Answer from the drawing. Dimensions are ordinates in mm from the lowest x, y and z of the part. A direction names the side the tool comes from. Round coordinates to 2 decimals unless told otherwise and drop trailing zeros. Order: outer loops, then holes, each group sorted by start corner. A loop starts at its lowest first (then second) coordinate and runs counter-clockwise, first axis right, second up. Notation, with made-up numbers: (88.25, 69) - (140.25, 69) arc R22 ccw to (140.25, 83) - close; hole circle Ø3 at (13, 16.25). An arc over 180 degrees is marked (long way). One line per question, with ' | ' between items. Start each with the question number.
1) Flat-ended cylindrical pins translate along their axes: pin 1 (13.5 mm diameter, centred on x = 349, z = 53.5, fed in from -Y); pin 2 (1.5 mm diameter, centred on x = 227, y = 19.5, fed in from -Z); pin 3 (2 mm diameter, centred on x = 191.5, z = 192.5, fed in from +Y). Find the tip coordinate at first contact, or state that the pin passes through.
2) The part is cut by section D-D, the plane x = 162. Give the vertices of the cut face in (y, z), plus the area to 3 significant figures.
3) The mould has two halves that part along Z. Classify the marked faces 3, 4 and 5: pulls with the +Z half, pulls with the -Z half, needs draft (parallel to the pull), parting line crosses it, or undercut.
4) The part is cut by section C-C, the plane z = 170.5. Give the vertices of the cut face in (x, y), plus the area to 3 significant figures.
5) For the marked faces 1 and 2, determine the directions among +Z, -Z, +X, -X, +Y, -Y from which every point of the face is accessible in a straight line to the end or side of a thin tool.
6) Straight lines are drawn through the part: line 1 (Z direction, x = 50, y = 14.5); line 2 (Z direction, x = 200, y = 20); line 3 (X direction, y = 15, z = 369). For each, find the intervals that lie inside material, in ascending order. Write a range as from..to.
7) The part is cut by section A-A, the plane y = 8.5. Give the vertices of the cut face in (x, z), plus the area to 3 significant figures.
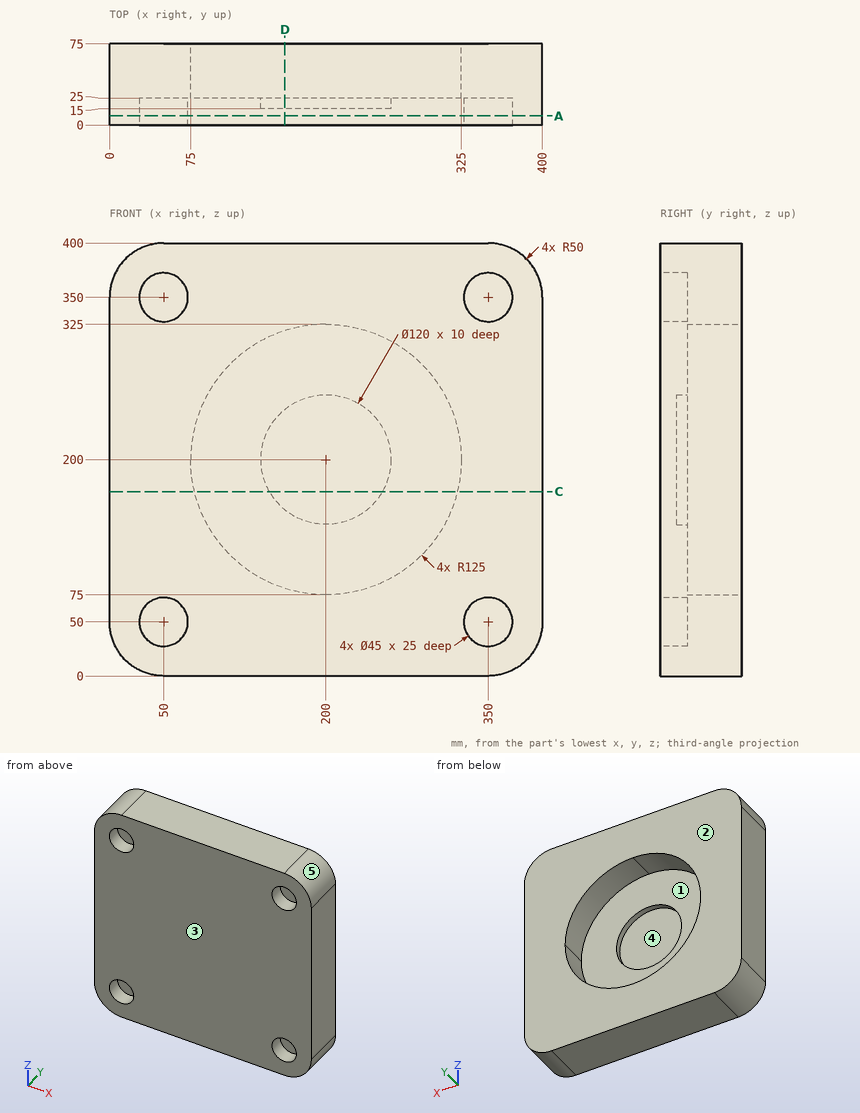
Values:
1) pin 1: stops at y = 25 | pin 2: stops at z = 0 | pin 3: stops at y = 15
2) outline: (0, 0) - (75, 0) - (75, 80.92) - (25, 80.92) - (25, 153.57) - (15, 153.57) - (15, 246.43) - (25, 246.43) - (25, 319.08) - (75, 319.08) - (75, 400) - (0, 400) - close | area: 17,200 mm^2
3) face 3: needs draft | face 4: undercut | face 5: pulls with the +Z half
4) outline: (0, 0) - (400, 0) - (400, 75) - (321.47, 75) - (321.47, 25) - (252.25, 25) - (252.25, 15) - (147.75, 15) - (147.75, 25) - (78.53, 25) - (78.53, 75) - (0, 75) - close | area: 16,800 mm^2
5) face 1: +Y | face 2: +Z, -Z, +X, -X, +Y
6) line 1: z = 0..27.5, 72.5..327.5, 372.5..400 | line 2: z = 0..140, 260..400 | line 3: x = 3.75..37.95, 62.05..337.95, 362.05..396.25
7) outline: (0, 50) arc R50 ccw to (50, 0) - (350, 0) arc R50 ccw to (400, 50) - (400, 350) arc R50 ccw to (350, 400) - (50, 400) arc R50 ccw to (0, 350) - close; hole circle Ø45 at (50, 50); hole circle Ø45 at (50, 350); hole circle Ø45 at (350, 50); hole circle Ø45 at (350, 350) | area: 151,000 mm^2
